```python
from build123d import *

# Parameters (mm, degrees)
BOSS_EXTRUDE1_DEPTH = 11.53
SKETCH2_R           = 1.5
CUT_EXTRUDE1_DEPTH  = 10


with BuildPart() as part:
    # Sketch1 → Boss-Extrude1 (new body)
    with BuildSketch(Plane(origin=(0, 0, 0), x_dir=(0, 0, -1), z_dir=(1, 0, 0))):
        with BuildLine():
            Line((-6.35, 5), (-11.155, 5))
            Line((-11.155, 5), (-11.155, -5))
            Line((-11.155, -5), (-6.155, -5))
            Line((-6.155, -5), (6.155, -5))
            Line((6.155, -5), (11.155, -5))
            Line((11.155, -5), (11.155, 5))
            Line((11.155, 5), (6.35, 5))
            ThreePointArc((6.35, 5), (0, -1.35), (-6.35, 5))
        make_face()
    extrude(amount=BOSS_EXTRUDE1_DEPTH)

    # Sketch2 → Cut-Extrude1 (cut)
    with BuildSketch(Plane(origin=(0, 5, 0), x_dir=(1, 0, 0), z_dir=(0, 1, 0))):
        with Locations((5.5, -8.655)):
            Circle(SKETCH2_R)
        with Locations((5.5, 8.655)):
            Circle(SKETCH2_R)
    extrude(amount=-CUT_EXTRUDE1_DEPTH, mode=Mode.SUBTRACT)


solid = part.part
```
Verification items for the finished model (mm, model axes). Give positions to 0.01 mm unless a question says otherwise; leave off trailing zeros. Order: outer loops, then holes, each group sorted by start corner. A loop starts at its lowest first (then second) coordinate and runs counter-clockwise, first axis right, second up. Notation, with made-up numbers: (47.25, 65.25) -> (95.25, 65.25) arc R31 ccw to (95.25, 89.25) -> close; hole circle Ø4 at (-14, 74). An arc over 180 degrees is marked (long way). Use a Markdown table: item, result.
1) Depth check by flat-ended pin: pin 1 Ø2.5 at (x, z) = (5.5, -8.655) entering from -Y; pin 2 Ø1.5 at (x, z) = (2, -4) entering from +Y; pin 3 Ø5 at (x, z) = (5.5, 8.655) entering from +Y. Enter the tip coordinate at first touch or a pass-through.
Results:
| item | result |
|---|---|
| pin 1 | through |
| pin 2 | y = 0.79 |
| pin 3 | y = 5 |
2) Material ranges on probe 1 along Z at (x, y) = (5.5, -2.5) (3 decimals); probe 2 along Z at (x, y) = (5.5, 0) (3 decimals); probe 3 along Z at (x, y) = (5.5, -0.25) (3 decimals), recorded low to high.
Results:
| item | result |
|---|---|
| probe 1 | -11.155 to -10.155, -7.155 to 7.155, 10.155 to 11.155 |
| probe 2 | -11.155 to -10.155, -7.155 to -3.914, 3.914 to 7.155, 10.155 to 11.155 |
| probe 3 | -11.155 to -10.155, -7.155 to -3.572, 3.572 to 7.155, 10.155 to 11.155 |
3) Mould release check, pull along X, two halves, no side actions. Record for faces 1 (the flat face through (11.53, -2, 0)), 2 (the flat face through (6, 0, 11.155)), 3 (the flat face through (0, -2, 0)), 4 (the cylindrical face through (5.3, 0.07, 7.17)): pulls with the +X half, pulls with the -X half, needs draft (parallel to the pull), parting line crosses it, or undercut.
Results:
| item | result |
|---|---|
| face 1 | pulls with the +X half |
| face 2 | needs draft |
| face 3 | pulls with the -X half |
| face 4 | undercut |
4) Section check C-C, the plane z = -9.5. Record the boundary of the cut face in (x, y), then the cut area to 3 significant figures.
Results:
| item | result |
|---|---|
| outline | (0, -5) -> (4.26, -5) -> (4.26, 5) -> (0, 5) -> close; (6.74, -5) -> (11.53, -5) -> (11.53, 5) -> (6.74, 5) -> close |
| area | 90.5 mm² |
5) Section check D-D, the plane y = -0.25. Record the boundary of the cut face in (x, z) (3 decimals), then the cut area to 3 significant figures.
Results:
| item | result |
|---|---|
| outline | (0, -11.155) -> (11.53, -11.155) -> (11.53, -3.572) -> (0, -3.572) -> close; (0, 3.572) -> (11.53, 3.572) -> (11.53, 11.155) -> (0, 11.155) -> close; hole circle Ø3 at (5.5, -8.655); hole circle Ø3 at (5.5, 8.655) |
| area | 161 mm² |
6) Section check B-B, the plane x = 5.5. Record the boundary of the cut face in (y, z) (3 decimals).
Results:
| item | result |
|---|---|
| outline | (-5, -11.155) -> (5, -11.155) -> (5, -10.155) -> (-5, -10.155) -> close; (-5, -7.155) -> (5, -7.155) -> (5, -6.35) arc R6.35 cw to (5, 6.35) -> (5, 7.155) -> (-5, 7.155) -> close; (-5, 10.155) -> (5, 10.155) -> (5, 11.155) -> (-5, 11.155) -> close |
7) Section check A-A, the plane y = 4.5. Record the boundary of the cut face in (x, z) (3 decimals), then the cut area to 3 significant figures.
Results:
| item | result |
|---|---|
| outline | (0, -11.155) -> (11.53, -11.155) -> (11.53, -6.33) -> (0, -6.33) -> close; (0, 6.33) -> (11.53, 6.33) -> (11.53, 11.155) -> (0, 11.155) -> close; hole circle Ø3 at (5.5, -8.655); hole circle Ø3 at (5.5, 8.655) |
| area | 97.1 mm² |
